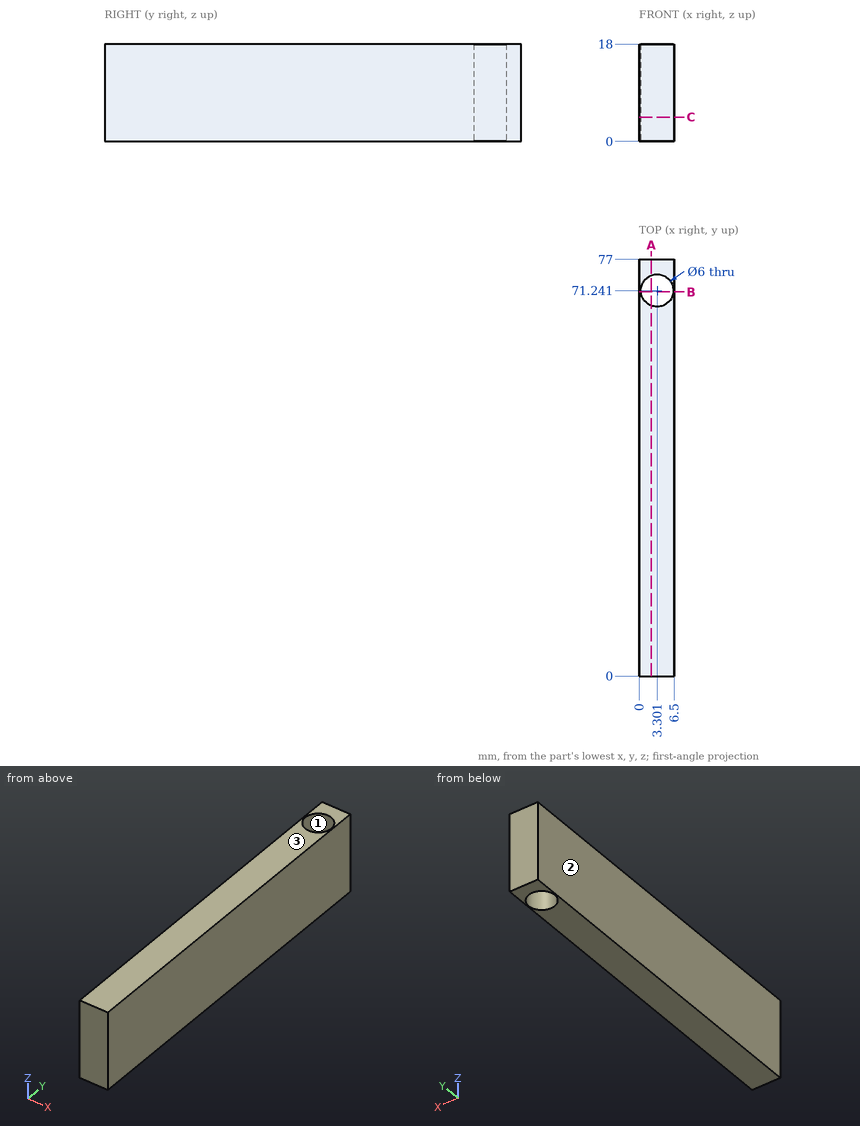
Here's the drawing with two shaded views (mm, measured from the low corner). I have some questions. Coordinates: 2 decimals unless noted, no trailing zeros. Loops run counter-clockwise (first coordinate to the right, second up) from the corner with the lowest first, then second, coordinate; pieces in that order, holes last.
Item 1: Suppose I cut it at B-B (y = 71). Please give me the cut outline in (x, z).
Answers below:
outline: (0, 0) - (0.31, 0) - (0.31, 18) - (0, 18) - close; (6.29, 0) - (6.5, 0) - (6.5, 18) - (6.29, 18) - close
Item 2: Please list where these lines run through material, in increasing order: L1, parallel to X at y = 71, z = 10.5; L2, parallel to Y at x = 3.5, z = 14.5 (1 decimal); L3, parallel to Y at x = 5.75, z = 10.5 (1 decimal).
Answers below:
L1: x = 0 to 0.31, 6.29 to 6.5
L2: y = 0 to 68.2, 74.2 to 77
L3: y = 0 to 69.5, 73 to 77
Item 3: If we mould it in two halves opening along X, with no side actions, what happens to the marked faces 1, 2 and 3? For each: released by +X, released by -X, zero draft, split by the parting line, or undercut.
Answers below:
face 1: undercut
face 2: released by -X
face 3: zero draft
Item 4: Suppose I cut it at C-C (z = 4.5). Please give me the cut outline in (x, y).
Answers below:
outline: (0, 0) - (6.5, 0) - (6.5, 77) - (0, 77) - close; hole circle Ø6 at (3.3, 71.24)
Item 5: Suppose I cut it at A-A (x = 2.25). Please give me the cut outline in (y, z).
Answers below:
outline: (0, 0) - (68.43, 0) - (68.43, 18) - (0, 18) - close; (74.05, 0) - (77, 0) - (77, 18) - (74.05, 18) - close
